```python
from build123d import *

# Parameters (mm, degrees)
F1_DEPTH = 3
F2_R     = 1.025
F2_R_2   = 3
F3_DEPTH = 25


with BuildPart() as f1:
    # F0 (on Top) → F1 (new body)
    with BuildSketch(Plane.XY):
        with BuildLine():
            ThreePointArc((0, 5), (1.464466, 1.464466), (5, 0))
            Line((5, 0), (75, 0))
            ThreePointArc((75, 0), (78.535534, 1.464466), (80, 5))
            Line((80, 5), (80, 75))
            ThreePointArc((80, 75), (78.535534, 78.535534), (75, 80))
            Line((75, 80), (5, 80))
            ThreePointArc((5, 80), (1.464466, 78.535534), (0, 75))
            Line((0, 75), (0, 5))
        make_face()
    extrude(amount=F1_DEPTH)

    # F2 (on face) → F3 (cut)
    with BuildSketch(Plane.XY.offset(3)):
        with Locations((40, 48.5)):
            Circle(F2_R)
        with Locations((40, 31.5)):
            Circle(F2_R)
        with Locations((62.5, 62.5)):
            Circle(F2_R_2)
        with Locations((40, 65.5)):
            Circle(F2_R)
        with Locations((40, 14.5)):
            Circle(F2_R)
        with Locations((62.5, 17.5)):
            Circle(F2_R_2)
        with Locations((17.5, 62.5)):
            Circle(F2_R_2)
        with Locations((17.5, 17.5)):
            Circle(F2_R_2)
    extrude(amount=-F3_DEPTH, mode=Mode.SUBTRACT)


solid = f1.part
```
Source: CAD feature listing. Evaluate the final solid. Frame: model axes, mm. Round coordinates to 2 decimals unless told otherwise and drop trailing zeros. Loops run counter-clockwise (first coordinate to the right, second up) from the corner with the lowest first, then second, coordinate; pieces in that order, holes last. Notation, with made-up numbers: M 69,-8 L 104,-8 A20 ccw 104,16 Z; hole C -6,-28.75 d8. An arc over 180 degrees is marked long. Use a Markdown table: item, result. Add a question column.
1. Cut plane D-D, the plane z = 1.7. State how many separate pieces and enclosed holes the cut face has, and give its area (3 significant figures).
2. Cut plane A-A, the plane x = 62.5. Output: boundary loops of the cut face in (y, z).
3. Cut plane C-C, the plane y = 31.5. Output: boundary loops of the cut face in (x, z) (3 decimals).
4. Pull-direction query (Y, two-part tool) for faces 1 (the cylindrical face through (79, 78, 1)), 2 (the flat face through (39, 41, 0)), 3 (the cylindrical face through (59.5, 17.6, 1.5)), 4 (the cylindrical face through (1, 2, 1)); classes: +Y half, -Y half, draft (parallel to the pull), parting line (faces both ways), or undercut.
5. Ray query, line 1 along Y through (x, z) = (17.5, 1.1); line 2 along Y through (x, z) = (40, 1.4) (3 decimals); line 3 along X through (y, z) = (66, 0.75). Return the intervals inside material, ascending. Write a range as [from, to].
Solution:
| question | item | result |
|---|---|---|
| 1 | separate pieces | 1 |
| 1 | enclosed holes | 8 |
| 1 | area | 6,250 mm2 |
| 2 | outline | M 0,0 L 14.5,0 L 14.5,3 L 0,3 Z; M 20.5,0 L 59.5,0 L 59.5,3 L 20.5,3 Z; M 65.5,0 L 80,0 L 80,3 L 65.5,3 Z |
| 3 | outline | M 0,0 L 38.975,0 L 38.975,3 L 0,3 Z; M 41.025,0 L 80,0 L 80,3 L 41.025,3 Z |
| 4 | face 1 | +Y half |
| 4 | face 2 | draft |
| 4 | face 3 | undercut |
| 4 | face 4 | -Y half |
| 5 | line 1 | y = [0, 14.5], [20.5, 59.5], [65.5, 80] |
| 5 | line 2 | y = [0, 13.475], [15.525, 30.475], [32.525, 47.475], [49.525, 64.475], [66.525, 80] |
| 5 | line 3 | x = [0, 39.11], [40.89, 80] |
